```python
from build123d import *

# Parameters (mm, degrees)
F0_W     = 200
F0_H     = 20
F1_DEPTH = 38
F2_R     = 21.793090142
F3_DEPTH = 90
F5_DEPTH = 10
F6_R     = 9.0643869575
F7_DEPTH = 30
F9_DEPTH = 500


with BuildPart() as f1:
    # F0 (on Right) → F1 (new body)
    with BuildSketch(Plane.YZ):
        with Locations((37.7075445842, -36.2104274062)):
            Rectangle(F0_W, F0_H)
    extrude(amount=F1_DEPTH)

    # F2 (on Right) → F3 (cut)
    with BuildSketch(Plane.YZ):
        with Locations((-26.4385696501, -50.3528229892)):
            Circle(F2_R)
    extrude(amount=F3_DEPTH, mode=Mode.SUBTRACT)

    # F4 (on Right) → F5 (cut)
    with BuildSketch(Plane.YZ):
        with BuildLine():
            ThreePointArc((11.2052927819, -30.0548411677), (13.8513494477, -26.4329954922), (14.787788926, -22.0463722944))
            ThreePointArc((14.787788926, -22.0463722944), (13.3069508893, -16.6036806846), (9.2726999384, -12.6615248637))
            ThreePointArc((9.2726999384, -12.6615248637), (6.5794975023, -21.7647944508), (11.2052927819, -30.0548411677))
        make_face()
        with BuildLine():
            ThreePointArc((9.2726999384, -12.6615248637), (13.3069508893, -16.6036806846), (14.787788926, -22.0463722944))
            ThreePointArc((14.787788926, -22.0463722944), (13.8513494477, -26.4329954922), (11.2052927819, -30.0548411677))
            ThreePointArc((11.2052927819, -30.0548411677), (19.8066220011, -32.6052268486), (27.8363086721, -28.6037941775))
            ThreePointArc((27.8363086721, -28.6037941775), (24.3564768067, -20.5394542894), (28.1950566672, -12.6395737651))
            ThreePointArc((28.1950566672, -12.6395737651), (18.7286864775, -8.1750752909), (9.2726999384, -12.6615248637))
        make_face()
        with BuildLine():
            ThreePointArc((11.2052927819, -30.0548411677), (6.5794975023, -21.7647944508), (9.2726999384, -12.6615248637))
            ThreePointArc((9.2726999384, -12.6615248637), (-6.6314854274, -23.2326830707), (11.2052927819, -30.0548411677))
        make_face()
        with BuildLine():
            ThreePointArc((42.792336068, -13.8019084932), (35.7285589591, -10.2711993263), (28.1950566672, -12.6395737651))
            ThreePointArc((28.1950566672, -12.6395737651), (30.2635700166, -16.2843509129), (30.9811221322, -20.4133056104))
            ThreePointArc((30.9811221322, -20.4133056104), (30.1678997374, -24.800045706), (27.8363086721, -28.6037941775))
            ThreePointArc((27.8363086721, -28.6037941775), (34.8911306198, -31.3144718481), (41.9464400799, -28.6050633204))
            ThreePointArc((41.9464400799, -28.6050633204), (38.534072164, -20.984324628), (42.792336068, -13.8019084932))
        make_face()
        with BuildLine():
            ThreePointArc((30.9811221322, -20.4133056104), (30.2635700166, -16.2843509129), (28.1950566672, -12.6395737651))
            ThreePointArc((28.1950566672, -12.6395737651), (24.3564768067, -20.5394542894), (27.8363086721, -28.6037941775))
            ThreePointArc((27.8363086721, -28.6037941775), (30.1678997374, -24.800045706), (30.9811221322, -20.4133056104))
        make_face()
        with BuildLine():
            ThreePointArc((56.6680879545, -21.5020179749), (51.9968309101, -13.5674704697), (42.792336068, -13.8019084932))
            ThreePointArc((42.792336068, -13.8019084932), (44.7488004803, -17.0479416086), (45.430340027, -20.7762103528))
            ThreePointArc((45.430340027, -20.7762103528), (44.5200498141, -25.0607318438), (41.9464400799, -28.6050633204))
            ThreePointArc((41.9464400799, -28.6050633204), (51.5369946086, -29.674841375), (56.6680879545, -21.5020179749))
        make_face()
        with BuildLine():
            ThreePointArc((45.430340027, -20.7762103528), (44.7488004803, -17.0479416086), (42.792336068, -13.8019084932))
            ThreePointArc((42.792336068, -13.8019084932), (38.534072164, -20.984324628), (41.9464400799, -28.6050633204))
            ThreePointArc((41.9464400799, -28.6050633204), (44.5200498141, -25.0607318438), (45.430340027, -20.7762103528))
        make_face()
    extrude(amount=F5_DEPTH, mode=Mode.SUBTRACT)

    # F6 (on Top) → F7 (cut)
    with BuildSketch(Plane.XY):
        with Locations((25.8594062179, -6.084471941)):
            Circle(F6_R)
    extrude(amount=-F7_DEPTH, mode=Mode.SUBTRACT)

    # F8 (on Front) → F9 (cut, symmetric)
    with BuildSketch(Plane.XZ):
        Polygon((-0.5932430504, -29.512187466), (3.8069577422, -25.6109777838), (-0.5932430504, -25.7017035037), align=None)
    extrude(amount=F9_DEPTH, both=True, mode=Mode.SUBTRACT)


solid = f1.part
```
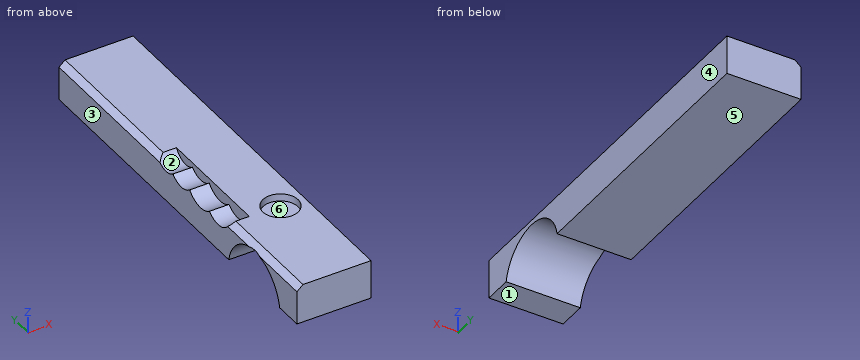
Here's how the part is built. I have some questions about the finished solid (model axes, mm). Face numbers are marked on the shaded views. A direction names the side the tool comes from. Coordinates: 2 decimals unless noted, no trailing zeros. Loops run counter-clockwise (first coordinate to the right, second up) from the corner with the lowest first, then second, coordinate; pieces in that order, holes last. Notation, with made-up numbers: (4, -21.75) - (44, -21.75) arc R24 ccw to (44, 11.25) - close; hole circle Ø5 at (-28, 21). An arc over 180 degrees is marked (long way). Return JSON: item names as keys, results as strings. Group by question number.
Item 1: On a 3-axis mill with a long thin cutter (end or side, diameter ignored), from which of +Z, -Z, +X, -X, +Y, -Y can I reach the whole of each face in a straight line? I mean the marked faces 1 and 2. Say none if no direction works.
Item 2: We'd pull the mould along X, two halves only. Please class the marked faces 3, 4, 5 and 6: +X half, -X half, draft (parallel to the pull), parting line (faces both ways), or undercut.
Item 3: If we section it at C-C on y = 51: Write out the boundary of the cut face in (x, z), and give its area (3 significant figures).
Item 4: I need wall thicknesses on line 1 (Z direction, x = 30.5, y = 0); line 2 (X direction, y = 23.5, z = -30); line 3 (Y direction, x = 9.5, z = -45.25). Which ranges of each line are inside material? Lowest first, please. Write a range as from..to.
Item 5: If we section it at D-D on x = 15: Write out the boundary of the cut face in (y, z).
Item 6: Will these pins go through, and if not, where does the flat tip stop? P1, Ø2, axis at y = 28.5, z = -28.5, coming from the -X side; P2, Ø5.5, axis at x = 24, y = -9, coming from the +Z side.
Item 7: If we section it at B-B on x = 31.5: Write out the boundary of the cut face in (y, z).
Item 8: If we section it at A-A on z = -34.75: Write out the boundary of the cut face in (x, y).
Calculated:
{
 "1": {"face 1": "-Z, +X, -X, +Y, -Y", "face 2": "+Z, -X"},
 "2": {"face 3": "-X half", "face 4": "+X half", "face 5": "draft", "face 6": "undercut"},
 "3": {"outline": "(0, -46.21) - (38, -46.21) - (38, -26.21) - (10, -26.21) - (10, -29.91) - (0, -29.91) - close", "area": "723 mm^2"},
 "4": {"line 1": "z = -46.21..-30", "line 2": "x = 10..38", "line 3": "y = -62.29..-47.63, -5.25..137.71"},
 "5": {"outline": "(-62.29, -46.21) - (-47.83, -46.21) arc R21.79 cw to (-5.04, -46.21) - (137.71, -46.21) - (137.71, -26.21) - (-62.29, -26.21) - close"},
 "6": {"P1": "stops at x = 0", "P2": "stops at z = -30"},
 "7": {"outline": "(-62.29, -46.21) - (-47.83, -46.21) arc R21.79 cw to (-5.04, -46.21) - (137.71, -46.21) - (137.71, -26.21) - (1.01, -26.21) - (1.01, -30) - (-13.18, -30) - (-13.18, -26.21) - (-62.29, -26.21) - close"},
 "8": {"outline": "(0, -62.29) - (38, -62.29) - (38, -41.65) - (0, -41.65) - close; (0, -11.22) - (38, -11.22) - (38, 137.71) - (0, 137.71) - close"}
}
